from build123d import *

# Parameters (mm, degrees)
F0_W     = 76.2
F0_H     = 76.2
F1_DEPTH = 76.2
F3_DEPTH = 25.4
F4_W     = 38.1
F4_H     = 38.1
F5_DEPTH = 25.4
F6_W     = 38.1
F6_H     = 38.1
F7_DEPTH = 25.4


with BuildPart() as f1:
    # F0 (on Front) → F1 (new body)
    with BuildSketch(Plane.XZ):
        with Locations((-38.1, 38.1)):
            Rectangle(F0_W, F0_H)
    extrude(amount=F1_DEPTH)

    # F2 (on face) → F3 (join)
    with BuildSketch(Plane.XZ.offset(76.2)):
        with BuildLine():
            Line((-38.1, 38.1), (-38.1, 57.15))
            ThreePointArc((-38.1, 57.15), (-51.570384, 51.570384), (-57.15, 38.1))
            Line((-57.15, 38.1), (-38.1, 38.1))
        make_face()
        with BuildLine():
            ThreePointArc((-57.15, 38.1), (-38.1, 19.05), (-19.05, 38.1))
            ThreePointArc((-19.05, 38.1), (-24.629616, 51.570384), (-38.1, 57.15))
            Line((-38.1, 57.15), (-38.1, 38.1))
            Line((-38.1, 38.1), (-57.15, 38.1))
        make_face()
    extrude(amount=F3_DEPTH)

    # F4 (on face) → F5 (join)
    with BuildSketch(Plane.YZ):
        with Locations((-38.1, 38.1)):
            Rectangle(F4_W, F4_H)
    extrude(amount=F5_DEPTH)

    # F6 (on face) → F7 (cut)
    with BuildSketch(Plane(origin=(0, 0, 0), x_dir=(1, 0, 0), z_dir=(0, 0, -1))):
        with Locations((-38.1, 38.1)):
            Rectangle(F6_W, F6_H)
    extrude(amount=-F7_DEPTH, mode=Mode.SUBTRACT)


solid = f1.part
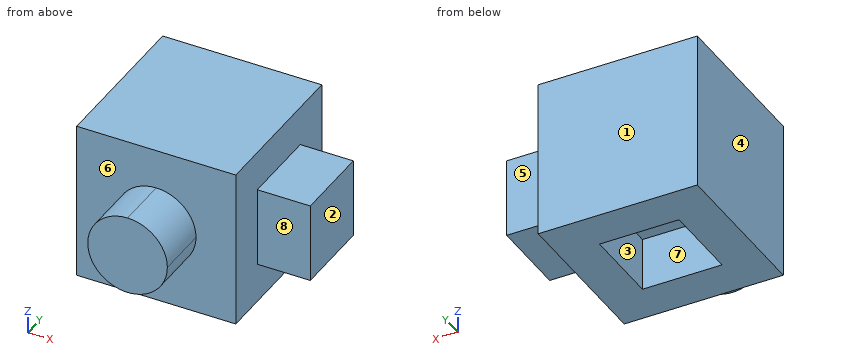
Geometry check sheet. Reference: the model listing, model coordinates, mm. Face numbers are marked on the shaded views. A direction names the side the tool comes from. Coordinates: 2 decimals unless noted, no trailing zeros. Order: outer loops, then holes, each group sorted by start corner. A loop starts at its lowest first (then second) coordinate and runs counter-clockwise, first axis right, second up. Notation, with made-up numbers: (11, 67.25) -> (54, 67.25) arc R22 cw to (54, 99.25) -> close; hole circle Ø11 at (74.5, 26.25). An arc over 180 degrees is marked (long way). Use a Markdown table: item, result. Add a question column.
1. Material ranges on L1, parallel to Y at x = -52, z = 16; L2, parallel to Z at x = 3, y = -22.5, recorded low to high.
2. Mould release check, pull along X, two halves, no side actions. Record for the marked faces 1, 2, 3 and 4: pulls with the +X half, pulls with the -X half, needs draft (parallel to the pull), parting line crosses it, or undercut.
3. Cross-section at D-D (z = 45). Enter the section's corners in (x, y), and give its area (3 significant figures).
4. Cross-section at A-A (z = 8.5). Enter the section's corners in (x, y).
5. Set-up check for the marked faces 5, 6, 7 and 8: record each of +Z, -Z, +X, -X, +Y, -Y from which the full face is reachable in a straight line by a thin tool's end or side.
6. Cross-section at C-C (y = -11). Enter the section's corners in (x, z).
7. Go/stop test with flat-tipped pins: pin 1 Ø7.5 at (x, z) = (-44.5, 14) entering from -Y; pin 2 Ø6 at (y, z) = (-81, 24.5) entering from -X; pin 3 Ø4 at (y, z) = (-62, 13) entering from +X. Record where each tip stops, or that it passes through.
8. Cross-section at B-B (x = -44). Enter the section's corners in (y, z).
Filled sheet:
| question | item | result |
|---|---|---|
| 1 | L1 | -76.2 to -57.15, -19.05 to 0 |
| 1 | L2 | 19.05 to 57.15 |
| 2 | face 1 | needs draft |
| 2 | face 2 | pulls with the +X half |
| 2 | face 3 | undercut |
| 2 | face 4 | pulls with the -X half |
| 3 | outline | (-76.2, -76.2) -> (-55.86, -76.2) -> (-55.86, -101.6) -> (-20.34, -101.6) -> (-20.34, -76.2) -> (0, -76.2) -> (0, -57.15) -> (25.4, -57.15) -> (25.4, -19.05) -> (0, -19.05) -> (0, 0) -> (-76.2, 0) -> close |
| 3 | area | 7,680 mm2 |
| 4 | outline | (-76.2, -76.2) -> (0, -76.2) -> (0, 0) -> (-76.2, 0) -> close; hole (-57.15, -57.15) -> (-19.05, -57.15) -> (-19.05, -19.05) -> (-57.15, -19.05) -> close |
| 5 | face 5 | +Z, -Z, +X, +Y |
| 5 | face 6 | -Y |
| 5 | face 7 | -Z |
| 5 | face 8 | +Z, -Z, +X, -Y |
| 6 | outline | (-76.2, 0) -> (0, 0) -> (0, 76.2) -> (-76.2, 76.2) -> close |
| 7 | pin 1 | y = -76.2 |
| 7 | pin 2 | x = -53.93 |
| 7 | pin 3 | x = 0 |
| 8 | outline | (-101.6, 19.99) -> (-76.2, 19.99) -> (-76.2, 0) -> (-57.15, 0) -> (-57.15, 25.4) -> (-19.05, 25.4) -> (-19.05, 0) -> (0, 0) -> (0, 76.2) -> (-76.2, 76.2) -> (-76.2, 56.21) -> (-101.6, 56.21) -> close |
